Here's how the part is built. I have some questions about the finished solid (model axes, mm). A direction names the side the tool comes from. Round coordinates to 2 decimals unless told otherwise and drop trailing zeros. Write each loop counter-clockwise with the first axis right and the second up, starting at its lowest first coordinate (ties: lowest second). Pieces come first, ordered by that corner, then holes. Notation, with made-up numbers: (78.25, 25) -> (96.25, 25) arc R24 cw to (96.25, 57) -> close; hole circle Ø8 at (43.5, 66). An arc over 180 degrees is marked (long way). Put each result on its own line as item: value. Start each with the question number.
1) Which directions (+Z, -Z, +X, -X, +Y, -Y) give clear straight access to the entire face, cutting with the end or side of a thin tool? Please do faces 4 (the flat face through (3.6, -11.4, 3)), 5 (the flat face through (7, -7, 0)).
2) Will these pins go through, and if not, where does the flat tip stop? P1, Ø5, axis at y = -12.5, z = 3, coming from the +X side; P2, Ø1, axis at x = 2, z = 2, coming from the -Y side; P3, Ø2, axis at y = -9.5, z = 5.5, coming from the -X side; P4, Ø1, axis at x = 13.5, z = 5.5, coming from the -Y side.
3) If I drill on line 1 along Y through (x, z) = (0, 7.75); line 2 along Y through (x, z) = (-2.5, 4); line 3 along Z through (x, y) = (3, -12.5), over which ranges is the centre line in solid material (lowest first)? Write a range as [from, to].
4) We'd pull the mould along X, two halves only. Please class faces 1 (the cylindrical face through (11.207, 3.529, 6.944)), 2 (the cylindrical face through (4.57, 7.167, 6.077)), 3 (the flat face through (-4, 8, 11.5)): released by +X, released by -X, zero draft, split by the parting line, or undercut.
5) I want a section at A-A, the plane y = 0. List the corners of the cut face in (x, z) for me, then the cut area to 4 significant figures.
6) I want a section at C-C, the plane z = 9.25. List the corners of the cut face in (x, y) for me, then the cut area to 3 significant figures.
from build123d import *

# Parameters (mm, degrees)
SCHIZZO1_R        = 17.5
ESTRUSIONE1_DEPTH = 3
SCHIZZO2_R        = 11.75
ESTRUSIONE2_DEPTH = 8.5
SCHIZZO3_R        = 8.5
ESTRUSIONE3_DEPTH = 28.290108098
SMUSSO1_SIZE      = 0.5


with BuildPart() as part:
    # Schizzo1 → Estrusione1 (new body)
    with BuildSketch(Plane.XY):
        Circle(SCHIZZO1_R)
    extrude(amount=ESTRUSIONE1_DEPTH)

    # Schizzo2 → Estrusione2 (add)
    with BuildSketch(Plane.XY.offset(3)):
        Circle(SCHIZZO2_R)
    extrude(amount=ESTRUSIONE2_DEPTH)

    # Schizzo3 → Estrusione3 (cut, through all)
    with BuildSketch(Plane.XY.offset(11.5)):
        Circle(SCHIZZO3_R)
    extrude(amount=-ESTRUSIONE3_DEPTH, mode=Mode.SUBTRACT)

    # Smusso1
    smusso1_edges = [part.edges().sort_by_distance(p)[0] for p in [
        (-8.5, 0, 0),
        (-17.5, 0, 0),
        (-11.75, 0, 11.5),
    ]]
    chamfer(smusso1_edges, length=SMUSSO1_SIZE)


solid = part.part
Findings:
1. face 4: +Z
1. face 5: -Z, +X, -X, +Y, -Y
2. P1: stops at x = 14.36
2. P2: stops at y = -17.44
2. P3: stops at x = -8.11
2. P4: passes through
3. line 1: y = [-11.75, -8.5], [8.5, 11.75]
3. line 2: y = [-11.48, -8.12], [8.12, 11.48]
3. line 3: z = [0, 3]
4. face 1: split by the parting line
4. face 2: undercut
4. face 3: zero draft
5. outline: (-17.5, 0.5) -> (-17, 0) -> (-9, 0) -> (-8.5, 0.5) -> (-8.5, 11.5) -> (-11.25, 11.5) -> (-11.75, 11) -> (-11.75, 3) -> (-17.5, 3) -> close; (8.5, 0.5) -> (9, 0) -> (17, 0) -> (17.5, 0.5) -> (17.5, 3) -> (11.75, 3) -> (11.75, 11) -> (11.25, 11.5) -> (8.5, 11.5) -> close
5. area: 108.5 mm2
6. outline: circle Ø23.5 at (0, 0); hole circle Ø17 at (0, 0)
6. area: 207 mm2
